```python
from build123d import *

# Parameters (mm, degrees)
SKETCH1_R           = 15
BOSS_EXTRUDE1_DEPTH = 1


with BuildPart() as part:
    # Sketch1 → Boss-Extrude1 (new body)
    with BuildSketch(Plane(origin=(0, 0, 0), x_dir=(1, 0, 0), z_dir=(0, 1, 0))):
        Circle(SKETCH1_R)
        with BuildLine():
            Line((-2, 11.22497216), (-2, 9.886859967))
            ThreePointArc((-2, 9.886859967), (-1.82596012, 9.507716194), (-1.425, 9.392516968))
            ThreePointArc((-1.425, 9.392516968), (0, 9.5), (1.425, 9.392516968))
            ThreePointArc((1.425, 9.392516968), (1.82596012, 9.507716194), (2, 9.886859967))
            Line((2, 9.886859967), (2, 11.22497216))
            ThreePointArc((2, 11.22497216), (2.187228379, 11.615066909), (2.608695652, 11.713014428))
            ThreePointArc((2.608695652, 11.713014428), (3.708203932, 11.412678196), (4.774258025, 11.00938056))
            ThreePointArc((4.774258025, 11.00938056), (5.057660104, 10.682407105), (4.979839104, 10.256763744))
            Line((4.979839104, 10.256763744), (4.193316491, 9.174208239))
            ThreePointArc((4.193316491, 9.174208239), (4.111262594, 8.765176409), (4.367933739, 8.436299832))
            ThreePointArc((4.367933739, 8.436299832), (5.583959897, 7.685661447), (6.673632173, 6.761111863))
            ThreePointArc((6.673632173, 6.761111863), (7.06572813, 6.618631549), (7.429384469, 6.823067229))
            Line((7.429384469, 6.823067229), (8.215907082, 7.905622735))
            ThreePointArc((8.215907082, 7.905622735), (8.596669963, 8.111165936), (8.995216257, 7.942674896))
            ThreePointArc((8.995216257, 7.942674896), (9.708203932, 7.053423028), (10.333607408, 6.100537513))
            ThreePointArc((10.333607408, 6.100537513), (10.370694331, 5.669430868), (10.05754893, 5.370820192))
            Line((10.05754893, 5.370820192), (8.784928608, 4.957320783))
            ThreePointArc((8.784928608, 4.957320783), (8.478122734, 4.674637153), (8.49246525, 4.257702899))
            ThreePointArc((8.49246525, 4.257702899), (9.035036905, 2.935661447), (9.373163684, 1.547191827))
            ThreePointArc((9.373163684, 1.547191827), (9.60662815, 1.201454611), (10.020996586, 1.153094718))
            Line((10.020996586, 1.153094718), (11.293616907, 1.566594126))
            ThreePointArc((11.293616907, 1.566594126), (11.722475811, 1.509075263), (11.945869987, 1.138503515))
            ThreePointArc((11.945869987, 1.138503515), (12, 0), (11.945869987, -1.138503515))
            ThreePointArc((11.945869987, -1.138503515), (11.722475811, -1.509075263), (11.293616907, -1.566594126))
            Line((11.293616907, -1.566594126), (10.020996586, -1.153094718))
            ThreePointArc((10.020996586, -1.153094718), (9.60662815, -1.201454611), (9.373163684, -1.547191827))
            ThreePointArc((9.373163684, -1.547191827), (9.035036905, -2.935661447), (8.49246525, -4.257702899))
            ThreePointArc((8.49246525, -4.257702899), (8.478122734, -4.674637153), (8.784928608, -4.957320783))
            Line((8.784928608, -4.957320783), (10.05754893, -5.370820192))
            ThreePointArc((10.05754893, -5.370820192), (10.370694331, -5.669430868), (10.333607408, -6.100537513))
            ThreePointArc((10.333607408, -6.100537513), (9.708203932, -7.053423028), (8.995216257, -7.942674896))
            ThreePointArc((8.995216257, -7.942674896), (8.596669963, -8.111165936), (8.215907082, -7.905622735))
            Line((8.215907082, -7.905622735), (7.429384469, -6.823067229))
            ThreePointArc((7.429384469, -6.823067229), (7.06572813, -6.618631549), (6.673632173, -6.761111863))
            ThreePointArc((6.673632173, -6.761111863), (5.583959897, -7.685661447), (4.367933739, -8.436299832))
            ThreePointArc((4.367933739, -8.436299832), (4.111262594, -8.765176409), (4.193316491, -9.174208239))
            Line((4.193316491, -9.174208239), (4.979839104, -10.256763744))
            ThreePointArc((4.979839104, -10.256763744), (5.057660104, -10.682407105), (4.774258025, -11.00938056))
            ThreePointArc((4.774258025, -11.00938056), (3.708203932, -11.412678196), (2.608695652, -11.713014428))
            ThreePointArc((2.608695652, -11.713014428), (2.187228379, -11.615066909), (2, -11.22497216))
            Line((2, -11.22497216), (2, -9.886859967))
            ThreePointArc((2, -9.886859967), (1.82596012, -9.507716194), (1.425, -9.392516968))
            ThreePointArc((1.425, -9.392516968), (0, -9.5), (-1.425, -9.392516968))
            ThreePointArc((-1.425, -9.392516968), (-1.82596012, -9.507716194), (-2, -9.886859967))
            Line((-2, -9.886859967), (-2, -11.22497216))
            ThreePointArc((-2, -11.22497216), (-2.187228379, -11.615066909), (-2.608695652, -11.713014428))
            ThreePointArc((-2.608695652, -11.713014428), (-3.708203932, -11.412678196), (-4.774258025, -11.00938056))
            ThreePointArc((-4.774258025, -11.00938056), (-5.057660104, -10.682407105), (-4.979839104, -10.256763744))
            Line((-4.979839104, -10.256763744), (-4.193316491, -9.174208239))
            ThreePointArc((-4.193316491, -9.174208239), (-4.111262594, -8.765176409), (-4.367933739, -8.436299832))
            ThreePointArc((-4.367933739, -8.436299832), (-5.583959897, -7.685661447), (-6.673632173, -6.761111863))
            ThreePointArc((-6.673632173, -6.761111863), (-7.06572813, -6.618631549), (-7.429384469, -6.823067229))
            Line((-7.429384469, -6.823067229), (-8.215907082, -7.905622735))
            ThreePointArc((-8.215907082, -7.905622735), (-8.596669963, -8.111165936), (-8.995216257, -7.942674896))
            ThreePointArc((-8.995216257, -7.942674896), (-9.708203932, -7.053423028), (-10.333607408, -6.100537513))
            ThreePointArc((-10.333607408, -6.100537513), (-10.370694331, -5.669430868), (-10.05754893, -5.370820192))
            Line((-10.05754893, -5.370820192), (-8.784928608, -4.957320783))
            ThreePointArc((-8.784928608, -4.957320783), (-8.478122734, -4.674637153), (-8.49246525, -4.257702899))
            ThreePointArc((-8.49246525, -4.257702899), (-9.035036905, -2.935661447), (-9.373163684, -1.547191827))
            ThreePointArc((-9.373163684, -1.547191827), (-9.60662815, -1.201454611), (-10.020996586, -1.153094718))
            Line((-10.020996586, -1.153094718), (-11.293616907, -1.566594126))
            ThreePointArc((-11.293616907, -1.566594126), (-11.722475811, -1.509075263), (-11.945869987, -1.138503515))
            ThreePointArc((-11.945869987, -1.138503515), (-12, 0), (-11.945869987, 1.138503515))
            ThreePointArc((-11.945869987, 1.138503515), (-11.722475811, 1.509075263), (-11.293616907, 1.566594126))
            Line((-11.293616907, 1.566594126), (-10.020996586, 1.153094718))
            ThreePointArc((-10.020996586, 1.153094718), (-9.60662815, 1.201454611), (-9.373163684, 1.547191827))
            ThreePointArc((-9.373163684, 1.547191827), (-9.035036905, 2.935661447), (-8.49246525, 4.257702899))
            ThreePointArc((-8.49246525, 4.257702899), (-8.478122734, 4.674637153), (-8.784928608, 4.957320783))
            Line((-8.784928608, 4.957320783), (-10.05754893, 5.370820192))
            ThreePointArc((-10.05754893, 5.370820192), (-10.370694331, 5.669430868), (-10.333607408, 6.100537513))
            ThreePointArc((-10.333607408, 6.100537513), (-9.708203932, 7.053423028), (-8.995216257, 7.942674896))
            ThreePointArc((-8.995216257, 7.942674896), (-8.596669963, 8.111165936), (-8.215907082, 7.905622735))
            Line((-8.215907082, 7.905622735), (-7.429384469, 6.823067229))
            ThreePointArc((-7.429384469, 6.823067229), (-7.06572813, 6.618631549), (-6.673632173, 6.761111863))
            ThreePointArc((-6.673632173, 6.761111863), (-5.583959897, 7.685661447), (-4.367933739, 8.436299832))
            ThreePointArc((-4.367933739, 8.436299832), (-4.111262594, 8.765176409), (-4.193316491, 9.174208239))
            Line((-4.193316491, 9.174208239), (-4.979839104, 10.256763744))
            ThreePointArc((-4.979839104, 10.256763744), (-5.057660104, 10.682407105), (-4.774258025, 11.00938056))
            ThreePointArc((-4.774258025, 11.00938056), (-3.708203932, 11.412678196), (-2.608695652, 11.713014428))
            ThreePointArc((-2.608695652, 11.713014428), (-2.187228379, 11.615066909), (-2, 11.22497216))
        make_face(mode=Mode.SUBTRACT)
    extrude(amount=BOSS_EXTRUDE1_DEPTH)


solid = part.part
```
Part model, mm, in its own coordinate system. Round coordinates to 2 decimals unless told otherwise and drop trailing zeros. Loops run counter-clockwise (first coordinate to the right, second up) from the corner with the lowest first, then second, coordinate; pieces in that order, holes last.
1. Flat gauge pin, fed straight in: pin 1 (10 mm diameter, centred on x = -1, z = -1, fed in from -Y). Where does the tip first touch, or does it go through?
Solutions:
pin 1: passes through
2. Two-plate mould, pull along X, no slides. Class faces 1 (the face through (9.72, 0.49, 7.04)), 2 (the face through (0, 0, 10)), 3 (the face through (-14.985, 0.493, -0.66)): pulls with the +X half, pulls with the -X half, needs draft (parallel to the pull), parting line crosses it, or undercut.
Solutions:
face 1: undercut
face 2: needs draft
face 3: parting line crosses it
3. Slice it at A-A (x = 0). Give the cut face in (y, z), and give its area (3 significant figures).
Solutions:
outline: (0, -15) - (1, -15) - (1, -9.5) - (0, -9.5) - close; (0, 9.5) - (1, 9.5) - (1, 15) - (0, 15) - close
area: 11.0 mm2
4. Drill centre lines: line 1 along Z through (x, y) = (8.75, 0.6); line 2 along X through (y, z) = (0.25, 11); line 3 along Z through (x, y) = (8.5, 0.6). Where is each one in solid material? Low to high.
Solutions:
line 1: z = -12.18 to -8.09, -4.94 to -3.7, 3.7 to 4.94, 8.09 to 12.18
line 2: x = -10.2 to -4.79, -2 to 2, 4.79 to 10.2
line 3: z = -12.36 to -8.1, -4.72 to -4.24, 4.24 to 4.72, 8.1 to 12.36
5. Slice it at C-C (z = -12.5). Give the cut face in (x, y), and give its area (3 significant figures).
Solutions:
outline: (-8.29, 0) - (8.29, 0) - (8.29, 1) - (-8.29, 1) - close
area: 16.6 mm2
6. Slice it at B-B (z = 0). Give the cut face in (x, y), and give its area (3 significant figures).
Solutions:
outline: (-15, 0) - (-12, 0) - (-12, 1) - (-15, 1) - close; (12, 0) - (15, 0) - (15, 1) - (12, 1) - close
area: 6.00 mm2
